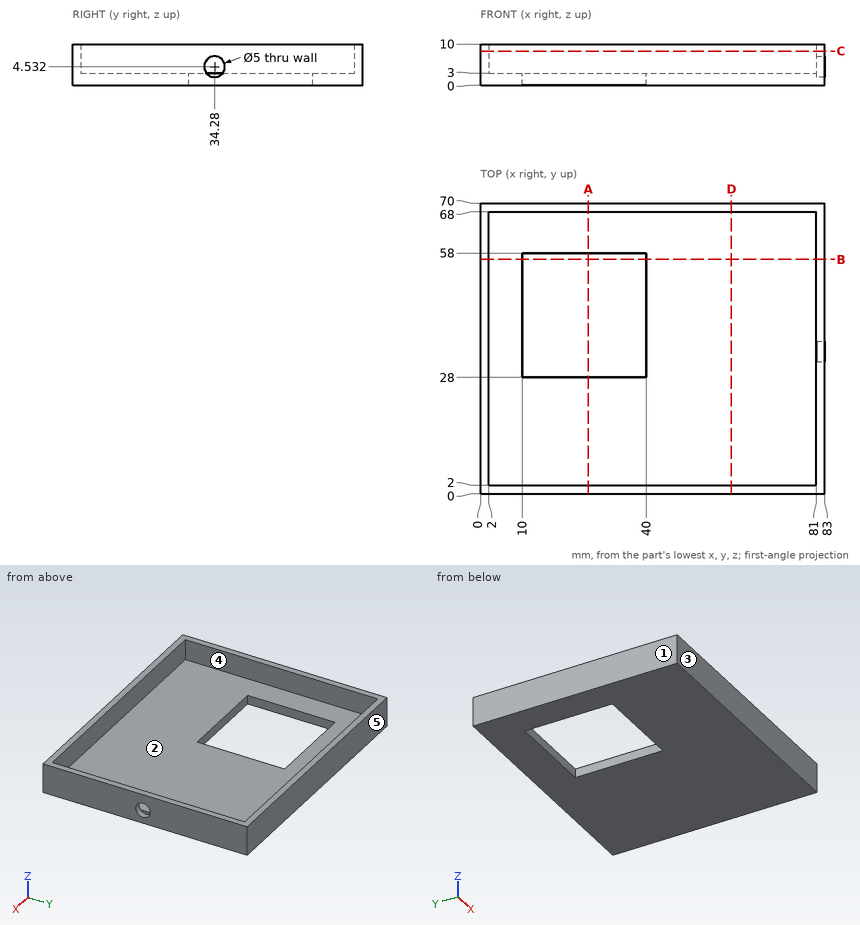
Print and shaded views of the part. All mm, measured from the part's lowest x, y and z. A direction names the side the tool comes from. Round coordinates to 2 decimals unless told otherwise and drop trailing zeros. Order: outer loops, then holes, each group sorted by start corner. A loop starts at its lowest first (then second) coordinate and runs counter-clockwise, first axis right, second up.
Q1. Wall check: L1, parallel to X at y = 44.5, z = 5.75; L2, parallel to Y at x = 19, z = 9; L3, parallel to X at y = 44.5, z = 1. Give the ranges that are in metal, low to high.
Q2. Two-plate mould, pull along Y, no slides. Class the marked faces 3, 4 and 5: pulls with the +Y half, pulls with the -Y half, needs draft (parallel to the pull), parting line crosses it, or undercut.
Q3. Slice it at B-B (y = 56.5). Write the cut outline in (x, z).
Q4. Drop flat-ended pins along their axis: pin 1 (4 mm diameter, centred on x = 32, y = 27, fed in from +Z); pin 2 (3 mm diameter, centred on y = 34.28, z = 4.53, fed in from +X); pin 3 (0.8 mm diameter, centred on y = 34, z = 2.5, fed in from +X). Give the stop position or say it passes through.
Q5. Slice it at C-C (z = 8.25). Write the cut outline in (x, y), and give its area (3 significant figures).
Q6. Which spindle directions (+Z, -Z, +X, -X, +Y, -Y) get a long thin tool onto all of the face, cutting with end or side? Do the marked faces 1 and 2. Say none if no direction does.
Q7. Slice it at A-A (x = 26). Write the cut outline in (y, z), and give its area (3 significant figures).
Q8. Slice it at D-D (x = 60.5). Write the cut outline in (y, z).
Results below:
1. L1: x = 0 to 2, 81 to 83
1. L2: y = 0 to 2, 68 to 70
1. L3: x = 0 to 10, 40 to 83
2. face 3: pulls with the -Y half
2. face 4: undercut
2. face 5: pulls with the +Y half
3. outline: (0, 0) - (10, 0) - (10, 3) - (2, 3) - (2, 10) - (0, 10) - close; (40, 0) - (83, 0) - (83, 10) - (81, 10) - (81, 3) - (40, 3) - close
4. pin 1: stops at z = 3
4. pin 2: stops at x = 2
4. pin 3: stops at x = 81
5. outline: (0, 0) - (83, 0) - (83, 70) - (0, 70) - close; hole (2, 2) - (81, 2) - (81, 68) - (2, 68) - close
5. area: 596 mm2
6. face 1: +Z, -Z, -X, +Y, -Y
6. face 2: +Z
7. outline: (0, 0) - (28, 0) - (28, 3) - (2, 3) - (2, 10) - (0, 10) - close; (58, 0) - (70, 0) - (70, 10) - (68, 10) - (68, 3) - (58, 3) - close
7. area: 148 mm2
8. outline: (0, 0) - (70, 0) - (70, 10) - (68, 10) - (68, 3) - (2, 3) - (2, 10) - (0, 10) - close
